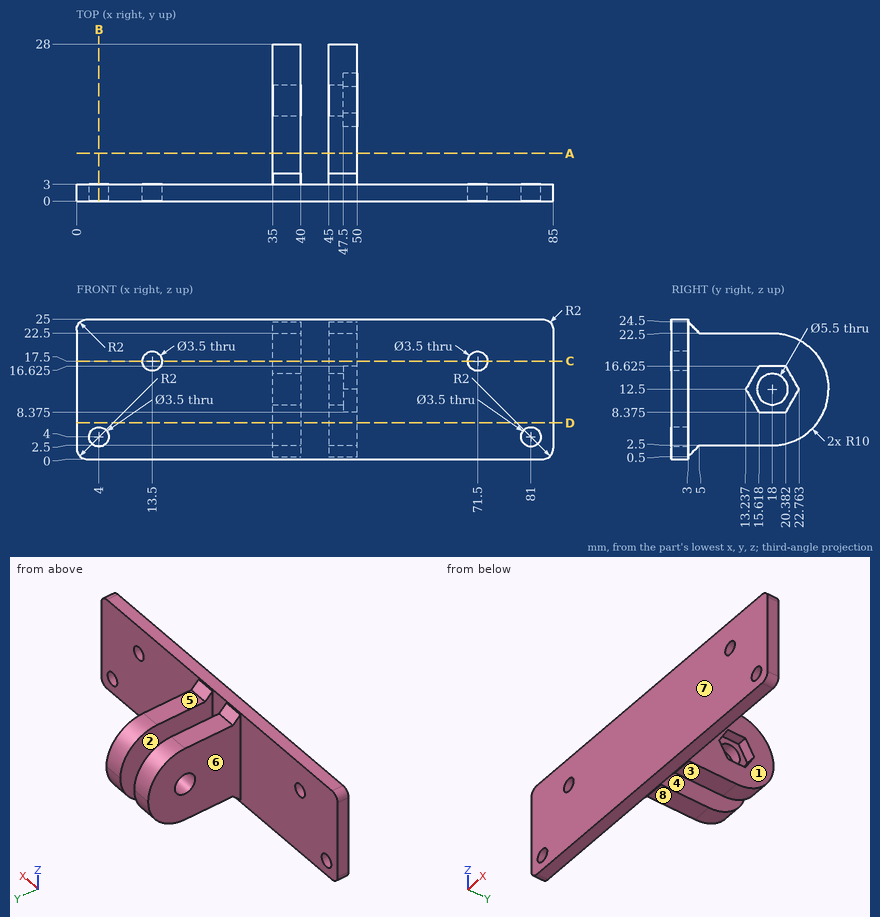
Verification items for this drawing (mm, ordinates from the low corner). A direction names the side the tool comes from. Give positions to 0.01 mm unless a question says otherwise; leave off trailing zeros. Write each loop counter-clockwise with the first axis right and the second up, starting at its lowest first coordinate (ties: lowest second). Pieces come first, ordered by that corner, then holes. Notation, with made-up numbers: M 84,79.25 L 137,79.25 A10 cw 137,83.25 Z; hole C -7.5,-24 d3. An arc over 180 degrees is marked long. Use one line per item in the form item = value.
(1) Section check C-C on z = 17.5. Record the boundary of the cut face in (x, y).
Answer block:
outline = M 0,0 L 11.75,0 L 11.75,3 L 0,3 Z; M 15.25,0 L 69.75,0 L 69.75,3 L 50,3 L 50,26.66 L 45,26.66 L 45,3 L 40,3 L 40,26.66 L 35,26.66 L 35,3 L 15.25,3 Z; M 73.25,0 L 85,0 L 85,3 L 73.25,3 Z
(2) Section check B-B on x = 4. Record the boundary of the cut face in (y, z), plus the area to 3 significant figures.
Answer block:
outline = M 0,0 L 3,0 L 3,2.25 L 0,2.25 Z; M 0,5.75 L 3,5.75 L 3,25 L 0,25 Z
area = 64.5 mm2
(3) Section check D-D on z = 6.5. Record the boundary of the cut face in (x, y), plus the area to 3 significant figures.
Answer block:
outline = M 0,0 L 85,0 L 85,3 L 50,3 L 50,26 L 45,26 L 45,3 L 40,3 L 40,26 L 35,26 L 35,3 L 0,3 Z
area = 485 mm2
(4) Draft check along X on the marked faces 1, 2 and 3. Enter one of: pulls with the +X half, pulls with the -X half, needs draft (parallel to the pull), parting line crosses it, or undercut.
Answer block:
face_1 = pulls with the +X half
face_2 = undercut
face_3 = needs draft
(5) Material ranges on line 1 along X through (y, z) = (2.15, 17.5); line 2 along X through (y, z) = (0.8, 4); line 3 along Z through (x, y) = (71.5, 0.75), recorded low to high.
Answer block:
line_1 = 0 to 11.75, 15.25 to 69.75, 73.25 to 85
line_2 = 0 to 2.25, 5.75 to 79.25, 82.75 to 85
line_3 = 0 to 15.75, 19.25 to 25
(6) Tool access check on the marked faces 4, 5, 6, 7 and 8. Record the directions out of +Z, -Z, +X, -X, +Y, -Y that give a thin tool (end or side, any length) a straight path to the whole face; none if there is none.
Answer block:
face_4 = +Z, -Z, +Y
face_5 = +Z, +X, -X, +Y
face_6 = +Z, -Z, -X, +Y
face_7 = +Z, -Z, +X, -X, -Y
face_8 = -Z, +X, -X, +Y
(7) Depth check by flat-ended pin: P1, Ø3, axis at y = 9.5, z = 22, coming from the +X side; P2, Ø12, axis at y = 10, z = 17, coming from the -X side; P3, Ø2.5, axis at x = 37.5, y = 10.5, coming from the +Z side; P4, Ø1.5, axis at x = 65.5, z = 14, coming from the -Y side. Enter the tip coordinate at first touch or a pass-through.
Answer block:
P1 = 50
P2 = 35
P3 = 22.5
P4 = 0
(8) Section check A-A on y = 8.5. Record the boundary of the cut face in (x, z), plus the area to 3 significant figures.
Answer block:
outline = M 35,2.5 L 40,2.5 L 40,22.5 L 35,22.5 Z; M 45,2.5 L 50,2.5 L 50,22.5 L 45,22.5 Z
area = 200 mm2
